The listing builds one solid part. Answer for the finished solid, in the listing's coordinates (mm). Face numbers are marked on the shaded views. A direction names the side the tool comes from. Give positions to 0.01 mm unless a question says otherwise; leave off trailing zeros. Order: outer loops, then holes, each group sorted by start corner. A loop starts at its lowest first (then second) coordinate and runs counter-clockwise, first axis right, second up. Notation, with made-up numbers: (51, 19) - (110, 19) arc R21 ccw to (110, 40) - close; hole circle Ø6 at (-33.75, -6). An arc over 180 degrees is marked (long way). Answer as a JSON object with one key per item and string values. Group by question number.
Q1. For the marked faces 3 and 4, determine the directions among +Z, -Z, +X, -X, +Y, -Y from which every point of the face is accessible in a straight line to the end or side of a thin tool.
Q2. The mould has two halves that part along Y. Classify the marked faces 1 and 2: released by +Y, released by -Y, zero draft, split by the parting line, or undercut.
Q3. Consider line 1 (X direction, y = 0, z = -11.65) (3 decimals); line 2 (X direction, y = 0, z = -3.25); line 3 (Z direction, x = -4.5, y = -2). Determine where each line is inside the solid, lowest interval first.
Q4. A cutting plane is placed at A-A, the plane z = 3.5. Give the vertices of the cut face in (x, y), and give its area (3 significant figures).
Q5. Given pin 1 (1 mm diameter, centred on x = -5, z = -9.5, fed in from -Y); pin 2 (7.5 mm diameter, centred on x = 0.5, y = -2.5, fed in from -Z); pin 3 (6 mm diameter, centred on y = -4.5, z = 4, fed in from +X); pin 4 (5 mm diameter, centred on x = 0, y = 0, fed in from -Z), each flat-ended and moving along its own axis, determine where each tip first touches the part or whether it passes through.
Q6. A cutting plane is placed at B-B, the plane z = -8.25. Give the vertices of the cut face in (x, y), and give its area (3 significant figures).
Autodesk Inventor part; units mm, degrees
ref_plane "YZ Plane" through (0, 0, 0) normal (1, 0, 0) x (0, 1, 0)
ref_plane "XZ Plane" through (0, 0, 0) normal (0, 1, 0) x (-1, 0, 0)
ref_plane "XY Plane" through (0, 0, 0) normal (0, 0, 1) x (1, 0, 0)
sketch "Sketch1" plane through (0, 0, 0) normal (1, 0, 0) x (0, 1, 0)
  line L0 (4, 11.492) -> (4, -11.492)
  line L1 (4, -11.492) -> (6.484, -11.492)
  line L2 (6.484, -11.492) -> (6.484, -12)
  line L3 (6.484, -12) -> (7.5, -12)
  line L4 (7.5, -12) -> (7.5, -8.75)
  line L5 (7.5, -8.75) -> (7.246, -8.75)
  line L6 (7.246, -8.75) -> (7.246, -7.5)
  line L7 (7.246, -7.5) -> (7.5, -7.5)
  line L8 (7.5, -7.5) -> (7.5, 7.5)
  line L9 (7.5, 7.5) -> (7.246, 7.5)
  line L10 (7.246, 7.5) -> (7.246, 8.75)
  line L11 (7.246, 8.75) -> (7.5, 8.75)
  line L12 (7.5, 8.75) -> (7.5, 12)
  line L13 (7.5, 12) -> (6.484, 12)
  line L14 (6.484, 12) -> (6.484, 11.492)
  line L15 (6.484, 11.492) -> (4, 11.492)
  line L16 (0, 0) -> (0, -1.7143)
  line L17 (4, 11.492) -> (4, 11.746)
  line L18 (4, 11.746) -> (4.762, 11.746)
  line L19 (4.762, 11.746) -> (4.762, 11.492)
  line L20 (4, -11.492) -> (4, -11.746)
  line L21 (4, -11.746) -> (4.762, -11.746)
  line L22 (4.762, -11.746) -> (4.762, -11.492)
  point P0 (4, 0)
  point P1 (7.5, 0)
  dimension "d0" = 8
  dimension "d1" = 15
  dimension "d2" = 24
  dimension "d3" = 1.016
  dimension "d4" = 0.254
  dimension "d5" = 0.762
  dimension "d6" = 0.508
  dimension "d7" = 1.25
  dimension "d8" = 0.254
  dimension "d9" = 15
revolve "Revolution1" add sketch "Sketch1" angle 360 about axis through (0, 0, 0) along (0, 0, -1)
chamfer "Chamfer1" distance 0.635 angle 45 2 edges at (0, -7.5, 12) (0, -7.5, -12)
properties part number "8mm Linear Bearing" material "Stainless Steel"
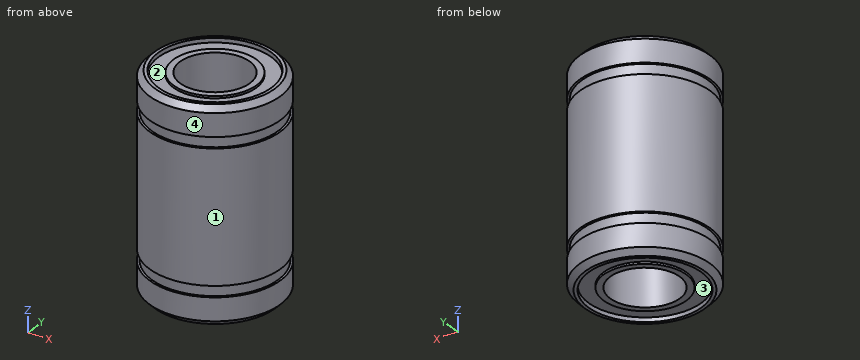
Reply:
{
 "1": {"face 3": "-Z", "face 4": "+Z, -Z"},
 "2": {"face 1": "split by the parting line", "face 2": "undercut"},
 "3": {"line 1": "x = -7.215 to -6.484, -4.762 to -4, 4 to 4.762, 6.484 to 7.215", "line 2": "x = -7.5 to -4, 4 to 7.5", "line 3": "z = -11.49 to 11.49"},
 "4": {"outline": "circle Ø15 at (0, 0); hole circle Ø8 at (0, 0)", "area": "126 mm^2"},
 "5": {"pin 1": "stops at y = -6", "pin 2": "stops at z = -11.75", "pin 3": "stops at x = 7.35", "pin 4": "passes through"},
 "6": {"outline": "circle Ø14.49 at (0, 0); hole circle Ø8 at (0, 0)", "area": "115 mm^2"}
}
